```python
from build123d import *

# Parameters (mm, degrees)
SKETCH1_W            = 158
SKETCH1_H            = 43.5
BOSS_EXTRUDE1_DEPTH  = 1.27
CUT_EXTRUDE1_DEPTH   = 159
M5_CLEARANCE_HOLE1_D = 5.3
CUT_EXTRUDE2_DEPTH   = 2.27


with BuildPart() as part:
    # Sketch1 → Boss-Extrude1 (new body)
    with BuildSketch(Plane(origin=(0, 0, 0), x_dir=(1, 0, 0), z_dir=(0, 1, 0))):
        Rectangle(SKETCH1_W, SKETCH1_H)
    extrude(amount=BOSS_EXTRUDE1_DEPTH)

    # Sketch2 → Cut-Extrude1 (cut, through all)
    with BuildSketch(Plane(origin=(79, 0, 0), x_dir=(0, 0, -1), z_dir=(1, 0, 0))):
        Polygon((-22.585561228, 12.404199387), (-22.585561228, -1.620794398), (-5.871224499, -1.620794398), align=None)
    extrude(amount=-CUT_EXTRUDE1_DEPTH, mode=Mode.SUBTRACT)

    # M5 Clearance Hole1 (through all)
    with Locations(Plane(origin=(0, 1.27, 0), x_dir=(1, 0, 0), z_dir=(0, 1, 0))):
        with Locations((-66.5, 8.639185421), (-20.5, 14.555407289), (20.5, 14.555407289), (66.5, 8.639185421)):
            Hole(M5_CLEARANCE_HOLE1_D / 2)

    # Sketch5 → Cut-Extrude2 (cut, through all)
    with BuildSketch(Plane.XZ):
        Polygon((-79, -13.288842768), (-64.136558606, 7.802812046), (-59.820077438, 13.928024129), (-79, 13.928024129), align=None)
        Polygon((64.136558606, 7.802812046), (59.820077438, 13.928024129), (79, 13.928024129), (79, -13.288842768), align=None)
    extrude(amount=-CUT_EXTRUDE2_DEPTH, mode=Mode.SUBTRACT)


solid = part.part
```
CAD build for the part. Positions are in the model's coordinates, mm. Round coordinates to 2 decimals unless told otherwise and drop trailing zeros. Write each loop counter-clockwise with the first axis right and the second up, starting at its lowest first coordinate (ties: lowest second). Pieces come first, ordered by that corner, then holes. Notation, with made-up numbers: (30.25, -1.5) -> (36.25, -1.5) arc R26 cw to (36.25, 35.5) -> close; hole circle Ø5 at (-8.5, 16.25). An arc over 180 degrees is marked (long way). Answer in a Markdown table with one row per item. Add a question column.
Item 1: Saw through at D-D, the plane x = 66.5. Write the cut outline in (y, z).
Item 2: Saw through at C-C, the plane x = -54. Write the cut outline in (y, z), then the cut area to 3 significant figures.
Item 3: Drill centre lines: line 1 (X direction, y = 0.4, z = -14.5); line 2 (Z direction, x = -20.5, y = 0.65); line 3 (Z direction, x = -66.5, y = 0.65). Where is each one in solid material? Low to high. Write a range as from..to.
Item 4: Drop a flat-ended pin along its axis: pin 1 Ø5 at (x, z) = (-66.5, -8.64) entering from +Y. Give the stop position or say it passes through.
Item 5: Mould opens along X. For faces 1 (the face through (-69.028, 0.626, -9.435)), 2 (the face through (-1, 0, -7)) say: pulls with the +X half, pulls with the -X half, needs draft (parallel to the pull), parting line crosses it, or undercut.
Item 6: Saw through at B-B, the plane y = 0.35. Write the cut outline in (x, z).
Item 7: Saw through at A-A, the plane x = -20.5. Write the cut outline in (y, z).
Findings below:
| question | item | result |
|---|---|---|
| 1 | outline | (0, -21.75) -> (1.27, -21.75) -> (1.27, -11.29) -> (0, -11.29) -> close; (0, -5.99) -> (1.27, -5.99) -> (1.27, 4.45) -> (0, 4.45) -> close |
| 2 | outline | (0, -21.75) -> (1.27, -21.75) -> (1.27, 9.32) -> (0, 7.8) -> close |
| 2 | area | 38.5 mm^2 |
| 3 | line 1 | x = -79..-23.15, -17.85..17.85, 23.15..79 |
| 3 | line 2 | z = -21.75..-17.21, -11.91..8.58 |
| 3 | line 3 | z = -21.75..-11.29, -5.99..4.45 |
| 4 | pin 1 | passes through |
| 5 | face 1 | undercut |
| 5 | face 2 | needs draft |
| 6 | outline | (-79, -21.75) -> (79, -21.75) -> (79, -13.29) -> (63.84, 8.22) -> (-63.84, 8.22) -> (-79, -13.29) -> close; hole circle Ø5.3 at (-66.5, -8.64); hole circle Ø5.3 at (-20.5, -14.56); hole circle Ø5.3 at (20.5, -14.56); hole circle Ø5.3 at (66.5, -8.64) |
| 7 | outline | (0, -21.75) -> (1.27, -21.75) -> (1.27, -17.21) -> (0, -17.21) -> close; (0, -11.91) -> (1.27, -11.91) -> (1.27, 9.32) -> (0, 7.8) -> close |
